```python
from build123d import *

# Parameters (mm, degrees)
PAD010_DEPTH = 3


with BuildPart() as part:
    # Sketch022 → Pad010 (new body, symmetric)
    with BuildSketch(Plane.XZ):
        with BuildLine():
            ThreePointArc((0.000532, 7.163), (-7.163, 0.000532), (-0.000532, -7.163))
            Line((-0.000532, -7.163), (538.329468, -7.203))
            ThreePointArc((538.329468, -7.203), (545.493, -0.040532), (538.330532, 7.123))
            Line((0.000532, 7.163), (538.330532, 7.123))
        make_face()
        with BuildLine():
            ThreePointArc((0.000458, 6.163), (-6.163, 0.000458), (-0.000458, -6.163))
            Line((-0.000458, -6.163), (538.329542, -6.203))
            ThreePointArc((538.329542, -6.203), (544.493, -0.040458), (538.330458, 6.123))
            Line((0.000458, 6.163), (538.330458, 6.123))
        make_face(mode=Mode.SUBTRACT)
    extrude(amount=PAD010_DEPTH, both=True)


solid = part.part
```
The model under review builds one solid part; all positions refer to its coordinate system, in mm. Round coordinates to 2 decimals unless told otherwise and drop trailing zeros. Loops run counter-clockwise (first coordinate to the right, second up) from the corner with the lowest first, then second, coordinate; pieces in that order, holes last. Notation, with made-up numbers: M 77,44 L 86,44 A33 cw 86,78 Z; hole C -12.5,-35 d6. An arc over 180 degrees is marked long. Answer as a JSON object with one key per item and string values.
(1) To check wall thickness, follow line 1 along Z through (x, y) = (378, 0.25); line 2 along Z through (x, y) = (122.5, -2.55); line 3 along X through (y, z) = (1.25, 0). State the ranges of each line that lie inside material, in increasing order.
Resolved:
{"line 1": "-7.19 to -6.19, 6.13 to 7.13", "line 2": "-7.17 to -6.17, 6.15 to 7.15", "line 3": "-7.16 to -6.16, 544.49 to 545.49"}
(2) Take a section at C-C on x = 73.5. Give the boundary of the cut face in (y, z), and give its area (3 significant figures).
Resolved:
{"outline": "M -3,-7.17 L 3,-7.17 L 3,-6.17 L -3,-6.17 Z; M -3,6.16 L 3,6.16 L 3,7.16 L -3,7.16 Z", "area": "12.0 mm²"}
(3) Take a section at B-B on z = 1. Give the boundary of the cut face in (x, y).
Resolved:
{"outline": "M -7.09,-3 L -6.08,-3 L -6.08,3 L -7.09,3 Z; M 544.4,-3 L 545.42,-3 L 545.42,3 L 544.4,3 Z"}
(4) Clearance check with flat-ended pins moving along their axes: P1, Ø3, axis at x = 369, y = -1, coming from the +Z side; P2, Ø2, axis at x = 173.5, y = 1, coming from the +Z side; P3, Ø2, axis at x = 280.5, y = 2, coming from the -Z side. State where each tip first meets the part, or that it passes through.
Resolved:
{"P1": "z = 7.14", "P2": "z = 7.15", "P3": "z = -7.18"}
(5) Take a section at A-A on y = -0.7. Give the boundary of the cut face in (x, z), and give its area (3 significant figures).
Resolved:
{"outline": "M 0,-7.16 L 538.33,-7.2 A7.16 ccw 538.33,7.12 L 0,7.16 A7.16 ccw Z; hole M 0,-6.16 L 538.33,-6.2 A6.16 ccw 538.33,6.12 L 0,6.16 A6.16 ccw Z", "area": "1,120 mm²"}
